```python
from build123d import *

# Parameters (mm, degrees)
BOSS_EXTRUDE1_DEPTH = 313.9694


with BuildPart() as part:
    # Sketch1 → Boss-Extrude1 (new body)
    with BuildSketch(Plane.XY):
        Polygon((-2.3876, 3.81), (2.3876, 3.81), (2.3876, -3.81), (3.9878, -3.81), (3.9878, 6.35), (0, 17.3609), (-3.9878, 6.35), (-3.9878, -3.81), (-2.3876, -3.81), align=None)
    extrude(amount=BOSS_EXTRUDE1_DEPTH)

    # Split1
    split(bisect_by=Plane(origin=(0, 142.217371243, 219.246784501), x_dir=(0, 0.8389556253011311, -0.5441998334946346), z_dir=(0, 0.5441998334946346, 0.8389556253011311)), keep=Keep.BOTTOM)

    # Split2
    split(bisect_by=Plane(origin=(0, 5.782993207, 8.915244702), x_dir=(0, -0.8389556253011311, 0.5441998334946346), z_dir=(0, -0.5441998334946346, -0.8389556253011311)), keep=Keep.BOTTOM)


solid = part.part
```
Input: part model. Units: mm. Frame: model coordinates. A direction names the side the tool comes from. Give positions to 0.01 mm unless a question says otherwise; leave off trailing zeros. Order: outer loops, then holes, each group sorted by start corner. A loop starts at its lowest first (then second) coordinate and runs counter-clockwise, first axis right, second up.
1. Cut plane B-B (y = -0.75). Return loops of the section in (x, z).
Computed:
outline: (-3.99, 13.15) - (-2.39, 13.15) - (-2.39, 311.98) - (-3.99, 311.98) - close; (2.39, 13.15) - (3.99, 13.15) - (3.99, 311.98) - (2.39, 311.98) - close
2. Draft query along X for faces 1 (the face through (-1.966, 11.933, 152.25)), 2 (the face through (3.988, 1, 159)), 3 (the face through (-0.06, 6.92, 8.18)), 4 (the face through (0, 3.81, 158)). Return one class per face: released by +X, released by -X, zero draft, split by the parting line, or undercut.
Computed:
face 1: released by -X
face 2: released by +X
face 3: zero draft
face 4: undercut
3. Cut plane A-A (z = 271). Return loops of the section in (x, y), and give its area (3 significant figures).
Computed:
outline: (-3.99, -3.81) - (-2.39, -3.81) - (-2.39, 3.81) - (2.39, 3.81) - (2.39, -3.81) - (3.99, -3.81) - (3.99, 6.35) - (0, 17.36) - (-3.99, 6.35) - close
area: 88.6 mm2
4. Pin query (flat end, axial travel): pin 1 Ø1.5 at (y, z) = (7.5, 79.5) entering from -X; pin 2 Ø1.5 at (x, y) = (2.5, 5) entering from -Z; pin 3 Ø4 at (x, y) = (-1, 3.5) entering from -Z. Return the tip coordinate at first contact, or that it passes through.
Computed:
pin 1: stops at x = -3.84
pin 2: stops at z = 8.94
pin 3: stops at z = 9.1
5. Line query: probe 1 along X at (y, z) = (-1.5, 165); probe 2 along Z at (x, y) = (-3.25, 4.75); probe 3 along X at (y, z) = (16, 213.5). Output: solid intervals per line, ascending.
Computed:
probe 1: x = -3.99 to -2.39, 2.39 to 3.99
probe 2: z = 9.59 to 308.42
probe 3: x = -0.49 to 0.49
6. Set-up query: faces 5 (the face through (-3.988, 1, 159)), 6 (the face through (-2.388, 0, 160)). Return all of +Z, -Z, +X, -X, +Y, -Y with unobstructed straight access to the full face (end or side cutting, diameter ignored); none if empty.
Computed:
face 5: +Z, -Z, -X, +Y, -Y
face 6: +Z, -Z, -Y
